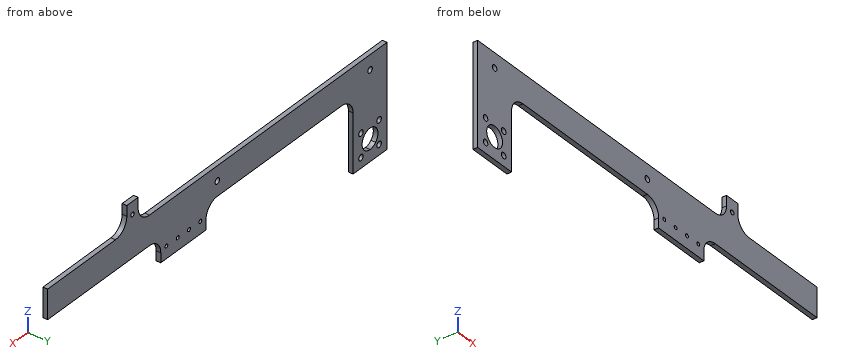
```python
from build123d import *

# Parameters (mm, degrees)
SKETCH1_R           = 2
SKETCH1_R_2         = 1.5
SKETCH1_R_3         = 1.25
BOSS_EXTRUDE1_DEPTH = 3.175
FILLET1_R           = 10
SKETCH2_W           = 70
SKETCH2_H           = 20
BOSS_EXTRUDE2_DEPTH = 3.175
FILLET2_R           = 10


with BuildPart() as part:
    # Sketch1 → Boss-Extrude1 (new body)
    with BuildSketch(Plane(origin=(0, 0, 0), x_dir=(1, 0, 0), z_dir=(0, 1, 0))):
        Polygon((220, -17), (225, -17), (230, -17), (230, 10), (230, 20), (200, 20), (200, 36.6), (195, 36.6), (160, 36.6), (160, 20), (30, 20), (30, 70), (15, 70), (0, 70), (0, 0), (220, 0), align=None)
        with Locations(Location((15, 10, 0), (0, 0, 270))):
            Circle(SKETCH1_R, mode=Mode.SUBTRACT)
        with Locations(Location((225, -8.5, 0), (0, 0, 270))):
            Circle(SKETCH1_R_2, mode=Mode.SUBTRACT)
        with BuildLine():
            ThreePointArc((148, 10), (150, 12), (152, 10))
            ThreePointArc((152, 10), (150, 8), (148, 10))
        make_face(mode=Mode.SUBTRACT)
        with Locations(Location((7, 47, 0), (0, 0, 270))):
            Circle(SKETCH1_R, mode=Mode.SUBTRACT)
        with Locations(Location((23, 47, 0), (0, 0, 270))):
            Circle(SKETCH1_R, mode=Mode.SUBTRACT)
        with BuildLine():
            ThreePointArc((10.050252532, 59.949747468), (12.321215973, 61.467156728), (15, 62))
            ThreePointArc((15, 62), (17.678784027, 48.532843272), (10.050252532, 59.949747468))
        make_face(mode=Mode.SUBTRACT)
        with Locations(Location((7, 63, 0), (0, 0, 270))):
            Circle(SKETCH1_R, mode=Mode.SUBTRACT)
        with Locations(Location((23, 63, 0), (0, 0, 270))):
            Circle(SKETCH1_R, mode=Mode.SUBTRACT)
        with Locations(Location((195, 28.3, 0), (0, 0, 270))):
            Circle(SKETCH1_R_3, mode=Mode.SUBTRACT)
        with Locations(Location((185, 28.3, 0), (0, 0, 270))):
            Circle(SKETCH1_R_3, mode=Mode.SUBTRACT)
        with Locations(Location((175, 28.3, 0), (0, 0, 270))):
            Circle(SKETCH1_R_3, mode=Mode.SUBTRACT)
        with Locations(Location((165, 28.3, 0), (0, 0, 270))):
            Circle(SKETCH1_R_3, mode=Mode.SUBTRACT)
    extrude(amount=BOSS_EXTRUDE1_DEPTH)

    # Fillet1
    fillet1_edges = [part.edges().sort_by_distance(p)[0] for p in [
        (200, 1.5875, -20),
        (220, 1.5875, 0),
        (30, 1.5875, -20),
        (160, 1.5875, -20),
    ]]
    fillet(fillet1_edges, radius=FILLET1_R)

    # Sketch2 → Boss-Extrude2 (add)
    with BuildSketch(Plane(origin=(0, 0, 0), x_dir=(-1, 0, 0), z_dir=(0, -1, 0))):
        with Locations((-265, 10)):
            Rectangle(SKETCH2_W, SKETCH2_H)
    extrude(amount=-BOSS_EXTRUDE2_DEPTH)

    # Fillet2
    fillet2_edges = [part.edges().sort_by_distance(p)[0] for p in [
        (230, 1.5875, 0),
    ]]
    fillet(fillet2_edges, radius=FILLET2_R)


solid = part.part
```
For this review, take the finished solid that the model builds, in its own axes (mm). Round coordinates to 2 decimals unless told otherwise and drop trailing zeros. Order: outer loops, then holes, each group sorted by start corner. A loop starts at its lowest first (then second) coordinate and runs counter-clockwise, first axis right, second up.
Q1. We need section A-A, the plane z = -55. Give the boundary of the cut face in (x, y) (3 decimals), plus the area to 3 significant figures.
Findings below:
outline: (0, 0) - (8, 0) - (8, 3.175) - (0, 3.175) - close; (22, 0) - (30, 0) - (30, 3.175) - (22, 3.175) - close
area: 50.8 mm2
Q2. We need section C-C, the plane x = 191. Give the boundary of the cut face in (y, z) (3 decimals).
Findings below:
outline: (0, -36.6) - (3.175, -36.6) - (3.175, 0) - (0, 0) - close
Q3. We need section B-B, the plane y = 0.75. State how many separate pieces and enclosed holes the cut face has, plus the area to 3 significant figures.
Findings below:
separate pieces: 1
enclosed holes: 12
area: 8,190 mm2
Q4. Wall thickness on line 1 (X direction, y = 2.2, z = -47); line 2 (X direction, y = 1.2, z = -30.5); line 3 (Z direction, x = 185, y = 0.75): over which ranges is each line inside the solid? List them lowest first.
Findings below:
line 1: x = 0 to 5, 9 to 21, 25 to 30
line 2: x = 0 to 30, 160 to 200
line 3: z = -36.6 to -29.55, -27.05 to 0
Q5. We need section D-D, the plane x = 255. Give the boundary of the cut face in (y, z) (3 decimals), plus the area to 3 significant figures.
Findings below:
outline: (0, -20) - (3.175, -20) - (3.175, 0) - (0, 0) - close
area: 63.5 mm2
Q6. Insertion check: P1, Ø1.5, axis at x = 167.5, y = 1.5, coming from the +Z side. The pin has a flat end and moves straight along its axis. Give the tip position at first contact, or say it passes through.
Findings below:
P1: stops at z = 0
